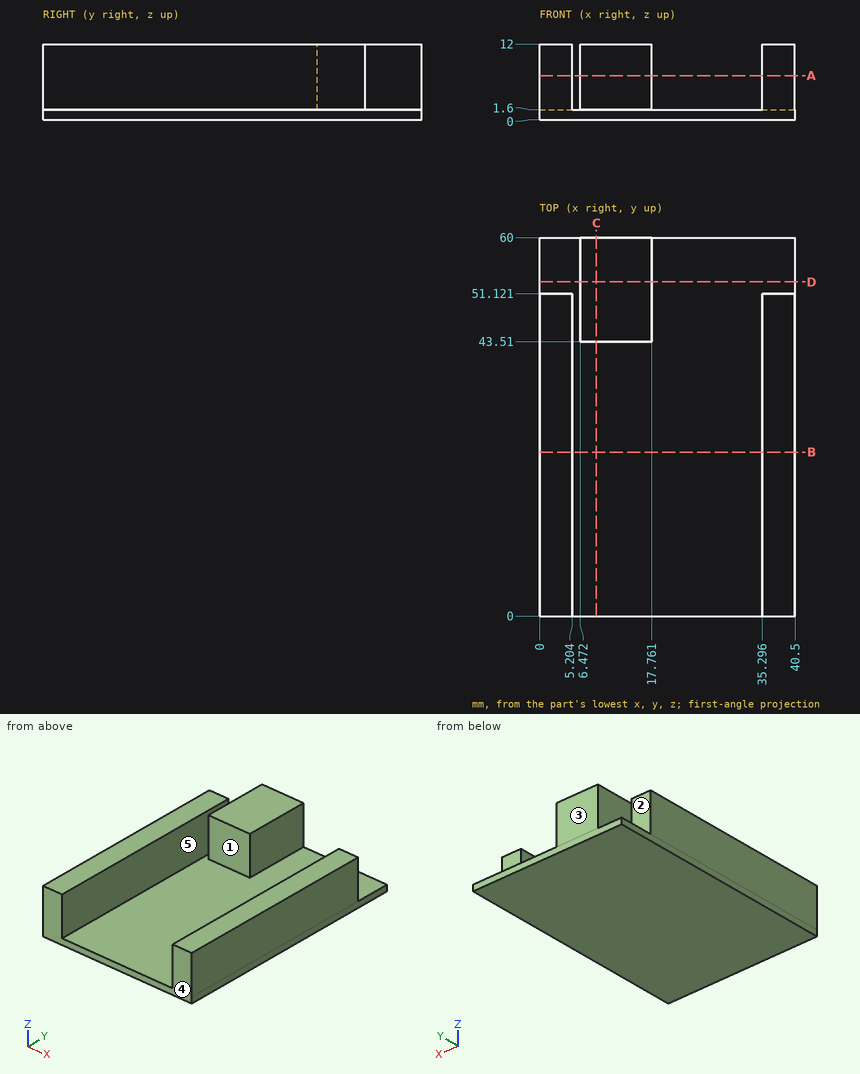
Job drawing, mm, ordinate dimensions from the low corner. One solid piece. A direction names the side the tool comes from. Round coordinates to 2 decimals unless told otherwise and drop trailing zeros. Loops run counter-clockwise (first coordinate to the right, second up) from the corner with the lowest first, then second, coordinate; pieces in that order, holes last.
Item 1: Drill centre lines: line 1 (X direction, y = 25, z = 9); line 2 (X direction, y = 50, z = 2); line 3 (Y direction, x = 37, z = 7.5). Where is each one in solid material? Low to high.
Item 2: Cut at A-A, the plane z = 7. Give the cut face in (x, y).
Item 3: Cut at C-C, the plane x = 9. Give the cut face in (y, z).
Item 4: 3-axis set-ups, long thin cutter, end or side, ignore diameter. For the marked faces 1, 2, 3, 4 and 5: which of +Z, -Z, +X, -X, +Y, -Y reach the whole face in a straight line?
Item 5: Cut at B-B, the plane y = 26. Give the cut face in (x, z).
Item 6: Cut at D-D, the plane y = 53. Give the cut face in (x, z).
Item 7: Drop flat-ended pins along their axis: P1, Ø12, axis at x = 16.5, y = 18.5, coming from the +Z side; P2, Ø2.5, axis at x = 37, z = 7.5, coming from the +Y side; P3, Ø5, axis at x = 14, z = 9.5, coming from the -Y side. Give the stop position or say it passes through.
A:
1. line 1: x = 0 to 5.2, 35.3 to 40.5
1. line 2: x = 0 to 5.2, 6.47 to 17.76, 35.3 to 40.5
1. line 3: y = 0 to 51.12
2. outline: (0, 0) - (5.2, 0) - (5.2, 51.12) - (0, 51.12) - close; (6.47, 43.51) - (17.76, 43.51) - (17.76, 60) - (6.47, 60) - close; (35.3, 0) - (40.5, 0) - (40.5, 51.12) - (35.3, 51.12) - close
3. outline: (0, 0) - (60, 0) - (60, 12) - (43.51, 12) - (43.51, 1.6) - (0, 1.6) - close
4. face 1: +Z, -Y
4. face 2: +Z, -X, +Y
4. face 3: +Z, -Z, +X, -X, +Y
4. face 4: +Z, -Z, +X, -X, -Y
4. face 5: +Z, +Y, -Y
5. outline: (0, 0) - (40.5, 0) - (40.5, 12) - (35.3, 12) - (35.3, 1.6) - (5.2, 1.6) - (5.2, 12) - (0, 12) - close
6. outline: (0, 0) - (40.5, 0) - (40.5, 1.6) - (17.76, 1.6) - (17.76, 12) - (6.47, 12) - (6.47, 1.6) - (0, 1.6) - close
7. P1: stops at z = 1.6
7. P2: stops at y = 51.12
7. P3: stops at y = 43.51
